Build history of the part. All positions in model axes, mm. A direction names the side the tool comes from. Round coordinates to 2 decimals unless told otherwise and drop trailing zeros. Loops run counter-clockwise (first coordinate to the right, second up) from the corner with the lowest first, then second, coordinate; pieces in that order, holes last. Notation, with made-up numbers: (34.5, 13) - (71.5, 13) arc R27 ccw to (71.5, 31) - close; hole circle Ø1 at (11.25, 76.25). An arc over 180 degrees is marked (long way). Put each result on its own line as item: value. Start each with the question number.
from build123d import *

# Parameters (mm, degrees)
SKETCH_2_W      = 20
SKETCH_2_H      = 20
SKETCH_2_R      = 2.1
EXTRUDE_1_DEPTH = 5
SKETCH_3_W      = 8
SKETCH_3_H      = 20
EXTRUDE_2_DEPTH = 5
FILLET_2_R      = 2
SKETCH_4_W      = 3
SKETCH_4_H      = 5.5
EXTRUDE_3_DEPTH = 3
CHAMFER_1_SIZE  = 1.5


with BuildPart() as part:
    # ｽｹｯﾁ2 → ﾎﾞｽ - 押し出し1 (new body)
    with BuildSketch(Plane.XY):
        Rectangle(SKETCH_2_W, SKETCH_2_H)
        Circle(SKETCH_2_R, mode=Mode.SUBTRACT)
    extrude(amount=EXTRUDE_1_DEPTH)

    # ｽｹｯﾁ3 → ﾎﾞｽ - 押し出し2 (add)
    with BuildSketch(Plane(origin=(10, 0, 0), x_dir=(0, 0, -1), z_dir=(1, 0, 0))):
        with Locations((-1, 0)):
            Rectangle(SKETCH_3_W, SKETCH_3_H)
    extrude(amount=EXTRUDE_2_DEPTH)

    # ﾌｨﾚｯﾄ2
    fillet_2_edges = [part.edges().sort_by_distance(p)[0] for p in [
        (15, 0, 5),
    ]]
    fillet(fillet_2_edges, radius=FILLET_2_R)

    # ｽｹｯﾁ4 → ﾎﾞｽ - 押し出し3 (add)
    with BuildSketch(Plane(origin=(0, 0, 0), x_dir=(-1, 0, 0), z_dir=(0, 0, -1))):
        with Locations((-8.5, 0)):
            Rectangle(SKETCH_4_W, SKETCH_4_H)
    extrude(amount=EXTRUDE_3_DEPTH)

    # 面取り1
    chamfer_1_edges = [part.edges().sort_by_distance(p)[0] for p in [
        (-2.1, 0, 5),
    ]]
    chamfer(chamfer_1_edges, length=CHAMFER_1_SIZE)


solid = part.part
Item 1: Slice it at C-C (z = -0.5). Give the cut face in (x, y).
Item 2: Drop flat-ended pins along their axis: pin 1 Ø1.5 at (y, z) = (-4.5, -1) entering from -X; pin 2 Ø1.5 at (y, z) = (5.5, 4) entering from +X; pin 3 Ø10 at (x, y) = (0.5, -4.5) entering from -Z. Give the stop position or say it passes through.
Item 3: Slice it at B-B (y = 0). Give the cut face in (x, z).
Item 4: Two-plate mould, pull along Y, no slides. Class faces 1 (the cylindrical face through (2.003, 0.631, 1.726)), 2 (the flat face through (2, -10, 2)), 3 (the flat face through (12, 0, -3)): pulls with the +Y half, pulls with the -Y half, needs draft (parallel to the pull), parting line crosses it, or undercut.
Item 5: Slice it at A-A (x = 0). Give the cut face in (y, z).
Item 6: Drill centre lines: probe 1 along Y at (x, z) = (0, 2.05); probe 2 along Z at (x, y) = (-7.75, -3); probe 3 along X at (y, z) = (8, -0.5). Where is each one in solid material? Low to high. Write a range as [from, to].
Item 7: Slice it at D-D (y = 4.75). Give the cut face in (x, z).
Item 8: Which spindle directions (+Z, -Z, +X, -X, +Y, -Y) get a long thin tool onto all of the face, cutting with end or side? Do faces 4 (the flat face through (10, -6, -1)), 5 (the flat face through (-10, 0, 2)), 6 (the cylindrical face through (14.4, 0.14, 4.43)), 7 (the flat face through (7, 0, -1)), 8 (the flat face through (9, 2.75, -1)). Say none if no direction does.
Computed values:
1. outline: (7, -2.75) - (10, -2.75) - (10, -10) - (15, -10) - (15, 10) - (10, 10) - (10, 2.75) - (7, 2.75) - close
2. pin 1: stops at x = 10
2. pin 2: stops at x = 14.98
2. pin 3: stops at z = 0
3. outline: (-10, 0) - (-2.1, 0) - (-2.1, 3.5) - (-3.6, 5) - (-10, 5) - close; (2.1, 0) - (7, 0) - (7, -3) - (15, -3) - (15, 3) arc R2 ccw to (13, 5) - (3.6, 5) - (2.1, 3.5) - close
4. face 1: undercut
4. face 2: pulls with the -Y half
4. face 3: needs draft
5. outline: (-10, 0) - (-2.1, 0) - (-2.1, 3.5) - (-3.6, 5) - (-10, 5) - close; (2.1, 0) - (10, 0) - (10, 5) - (3.6, 5) - (2.1, 3.5) - close
6. probe 1: y = [-10, -2.1], [2.1, 10]
6. probe 2: z = [0, 5]
6. probe 3: x = [10, 15]
7. outline: (-10, 0) - (10, 0) - (10, -3) - (15, -3) - (15, 3) arc R2 ccw to (13, 5) - (-10, 5) - close
8. face 4: -Z, -X, -Y
8. face 5: +Z, -Z, -X, +Y, -Y
8. face 6: +Z, +X, +Y, -Y
8. face 7: -Z, -X, +Y, -Y
8. face 8: -Z, -X, +Y
